Geometry: see drawing. Coordinates: mm, zero at the bounding-box minimum. Give positions to 0.01 mm unless a question says otherwise; leave off trailing zeros. Write each loop counter-clockwise with the first axis right and the second up, starting at its lowest first coordinate (ties: lowest second). Pieces come first, ordered by that corner, then holes. Notation, with made-up numbers: (1.25, -15) - (35.25, -15) arc R21 ccw to (35.25, -7) - close; hole circle Ø8 at (45.5, 12.25). An arc over 180 degrees is marked (long way). Use a Markdown table: item, result. Add a question column.
1. Section query D-D, the plane z = 40.5. Return loops of the section in (x, y) (1 decimal).
2. Section query C-C, the plane y = 10.75. Return loops of the section in (x, z) (1 decimal).
3. Pin query (flat end, axial travel): pin 1 (3 mm diameter, centred on x = 5.9, z = 37.83, fed in from -Y); pin 2 (3 mm diameter, centred on x = 54.1, z = 22.17, fed in from +Y); pin 3 (2 mm diameter, centred on x = 5.9, z = 22.17, fed in from +Y) (1 decimal); pin 4 (1 mm diameter, centred on y = 3.5, z = 8, fed in from +X). Return the tip coordinate at first contact, or that it passes through.
4. Section query A-A, the plane x = 30. Count the separate pieces of the cut face and the enclosed holes in it, plus the area to 3 significant figures.
5. Material intervals for probe 1 along X at (y, z) = (4.5, 9.5) (1 decimal); probe 2 along Y at (x, z) = (7, 44); probe 3 along X at (y, z) = (9.75, 37.5) (1 decimal), sorted ascending.
6. Mould query, pull axis Z, two halves, no side actions, for the marked faces 1, 2, 3 and 4. Classes: released by +Z, released by -Z, zero draft, split by the parting line, or undercut.
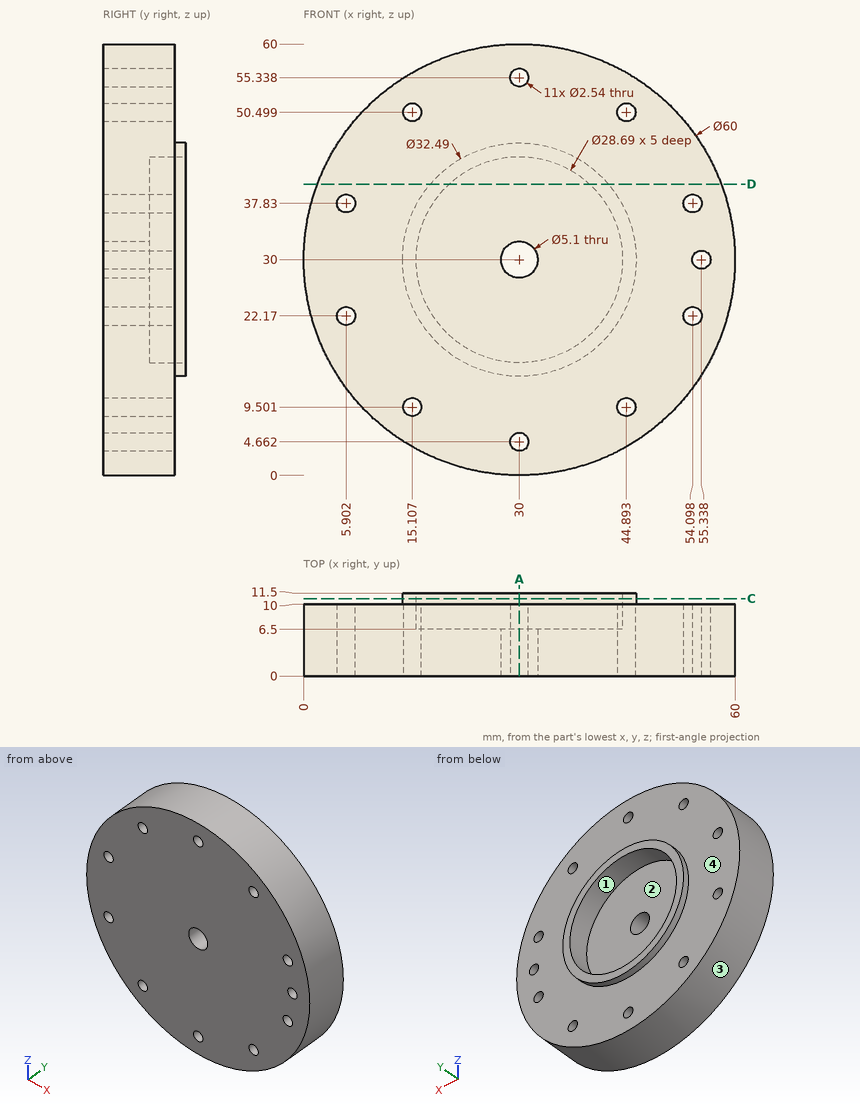
Result sheet:
| question | item | result |
|---|---|---|
| 1 | outline | (1.9, 0) - (58.1, 0) - (58.1, 10) - (42.4, 10) - (42.4, 11.5) - (39.8, 11.5) - (39.8, 6.5) - (20.2, 6.5) - (20.2, 11.5) - (17.6, 11.5) - (17.6, 10) - (1.9, 10) - close |
| 2 | outline | circle Ø32.5 at (30, 30); hole circle Ø28.7 at (30, 30) |
| 3 | pin 1 | stops at y = 0 |
| 3 | pin 2 | stops at y = 10 |
| 3 | pin 3 | passes through |
| 3 | pin 4 | stops at x = 50.92 |
| 4 | separate pieces | 4 |
| 4 | enclosed holes | 0 |
| 4 | area | 421 mm² |
| 5 | probe 1 | x = 8.1 to 13.8, 16.4 to 43.6, 46.2 to 51.9 |
| 5 | probe 2 | y = 0 to 10 |
| 5 | probe 3 | x = 1 to 4.7, 7.1 to 17.8, 42.2 to 52.9, 55.3 to 59 |
| 6 | face 1 | undercut |
| 6 | face 2 | undercut |
| 6 | face 3 | split by the parting line |
| 6 | face 4 | zero draft |
